Study the drawing (mm; zero at the part's minimum x, y, z) and answer. Give positions to 0.01 mm unless a question says otherwise; leave off trailing zeros.
Item 1: Find the intervals of material crossed by line 1 along Y through (x, z) = (38.1, 4.75); line 2 along Y through (x, z) = (67, 6.75) (1 decimal); line 3 along Z through (x, y) = (32, 2), in increasing order.
Item 2: A cutting plane is placed at A-A (y = 25.4). State how many separate pieces and enclosed holes the cut face has, plus the area to 3 significant figures.
Item 3: Given pin 1 Ø1.8 at (x, y) = (1.59, 25.4) entering from -Z; pin 2 Ø1 at (y, z) = (28, 7.5) entering from +X (1 decimal); pin 3 Ø1 at (x, z) = (40.5, 7) entering from +Y (1 decimal); pin 4 Ø0.6 at (y, z) = (33, 7) entering from -X (1 decimal), each flat-ended and moving along its own axis, determine where each tip first touches the part or whether it passes through.
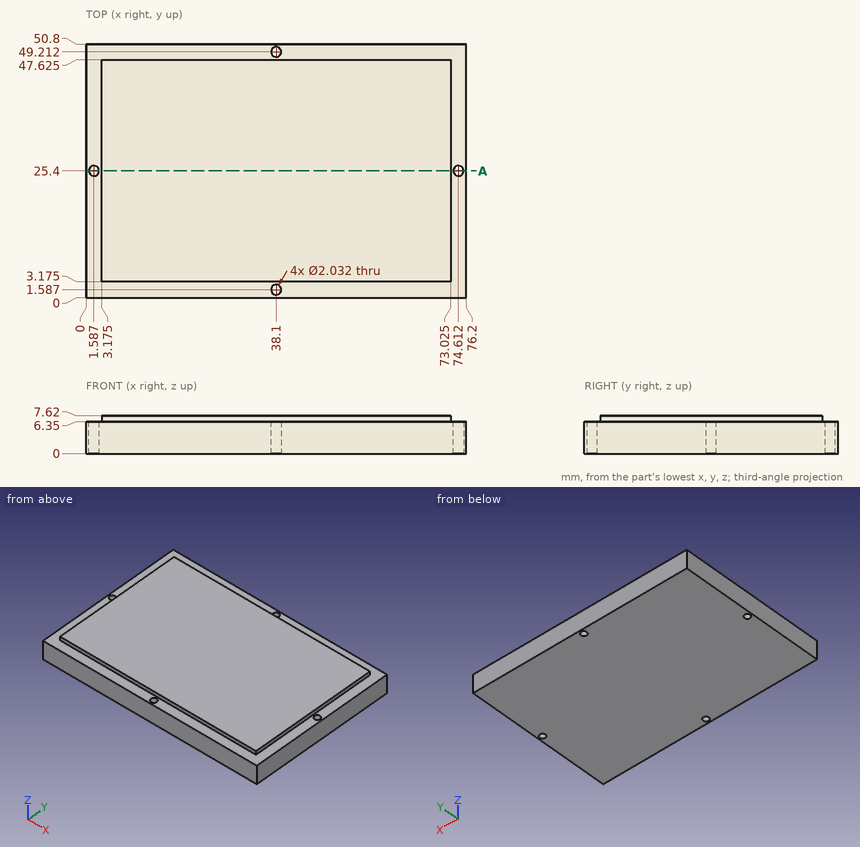
Response values:
1. line 1: y = 0 to 0.57, 2.6 to 48.2, 50.23 to 50.8
1. line 2: y = 3.2 to 47.6
1. line 3: z = 0 to 6.35
2. separate pieces: 3
2. enclosed holes: 0
2. area: 547 mm2
3. pin 1: passes through
3. pin 2: stops at x = 73
3. pin 3: stops at y = 47.6
3. pin 4: stops at x = 3.2
